The figure shows three views and two pictorial views of one solid part (mm, origin at its lowest corner). Answer the questions. Coordinates: 2 decimals unless noted, no trailing zeros. Write each loop counter-clockwise with the first axis right and the second up, starting at its lowest first coordinate (ties: lowest second). Pieces come first, ordered by that corner, then holes. Notation, with made-up numbers: M 57,-38.75 L 61,-38.75 A21 cw 61,-24.75 Z; hole C -32,-6.5 d1. An arc over 180 degrees is marked long. Answer as CSV lines item,"result".
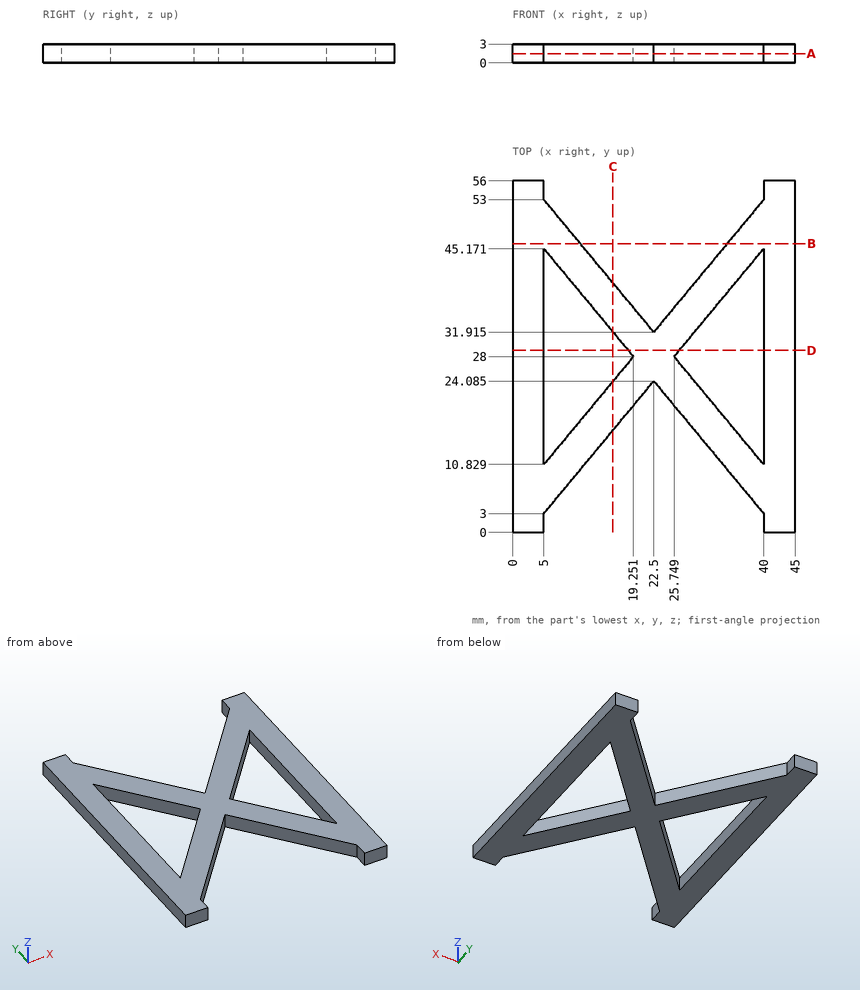
Q1. Straight lines are drawn through the part: line 1 (X direction, y = 14, z = 2.4); line 2 (X direction, y = 30, z = 1.55); line 3 (X direction, y = 25.5, z = 2.1) (1 decimal). For each, find the intervals that lie inside material, in ascending order.
Output:
line 1,"0 to 5, 7.63 to 14.13, 30.87 to 37.37, 40 to 45"
line 2,"0 to 5, 17.59 to 27.41, 40 to 45"
line 3,"0 to 5, 17.2 to 27.8, 40 to 45"
Q2. Find section C-C (x = 16). Give the vertices of the cut face in (y, z).
Output:
outline,"M 16.25,0 L 24.08,0 L 24.08,3 L 16.25,3 Z; M 31.92,0 L 39.75,0 L 39.75,3 L 31.92,3 Z"
Q3. Flat-ended cylindrical pins translate along their axes: pin 1 Ø1.5 at (y, z) = (1.5, 2) entering from -X; pin 2 Ø1 at (x, z) = (29, 2.5) entering from -Y. Find the tip coordinate at first contact, or state that the pin passes through.
Output:
pin 1,"x = 0"
pin 2,"y = 15.65"
Q4. Find section B-B (y = 46). Give the vertices of the cut face in (x, z).
Output:
outline,"M 0,0 L 10.81,0 L 10.81,3 L 0,3 Z; M 34.19,0 L 45,0 L 45,3 L 34.19,3 Z"
Q5. Find section A-A (z = 1.45). Give the vertices of the cut face in (x, y) (1 decimal).
Output:
outline,"M 0,0 L 5,0 L 5,3 L 22.5,24.1 L 40,3 L 40,0 L 45,0 L 45,56 L 40,56 L 40,53 L 22.5,31.9 L 5,53 L 5,56 L 0,56 Z; hole M 5,10.8 L 19.3,28 L 5,45.2 Z; hole M 25.7,28 L 40,10.8 L 40,45.2 Z"
Q6. Find section D-D (y = 29). Give the vertices of the cut face in (x, z).
Output:
outline,"M 0,0 L 5,0 L 5,3 L 0,3 Z; M 18.42,0 L 26.58,0 L 26.58,3 L 18.42,3 Z; M 40,0 L 45,0 L 45,3 L 40,3 Z"
